Geometry check sheet. Reference: the model listing, model coordinates, mm. A direction names the side the tool comes from. Round coordinates to 2 decimals unless told otherwise and drop trailing zeros. Order: outer loops, then holes, each group sorted by start corner. A loop starts at its lowest first (then second) coordinate and runs counter-clockwise, first axis right, second up.
```python
from build123d import *

# Parameters (mm, degrees)
BOSS_EXTRU_1_DEPTH  = 31.5
ESQUISSE3_R         = 3.5
BOSS_EXTRU_2_DEPTH  = 3
ESQUISSE5_R         = 2
BOSS_EXTRU_3_DEPTH  = 0.5
ESQUISSE6_R         = 2.5
BOSS_EXTRU_4_DEPTH  = 4.5
ESQUISSE8_R         = 2
BOSS_EXTRU_5_DEPTH  = 0.5
ESQUISSE9_R         = 2.5
BOSS_EXTRU_6_DEPTH  = 1
CHANFREIN1_SIZE     = 0.5
ESQUISSE10_R        = 5
BOSS_EXTRU_7_DEPTH  = 2
ESQUISSE11_R        = 3
BOSS_EXTRU_8_DEPTH  = 1
ESQUISSE13_R        = 3.375
BOSS_EXTRU_9_DEPTH  = 5
ESQUISSE15_R        = 3
BOSS_EXTRU_10_DEPTH = 0.5
ESQUISSE16_R        = 3.375
BOSS_EXTRU_11_DEPTH = 6.5


with BuildPart() as part:
    # Esquisse1 → Boss.-Extru.1 (new body)
    with BuildSketch(Plane(origin=(0, 0, 0), x_dir=(1, 0, 0), z_dir=(0, 1, 0))):
        with BuildLine():
            Line((1.18016373, -3.5), (1.18016373, -7.912472027))
            ThreePointArc((1.18016373, -7.912472027), (5.676756903, -5.636881324), (7.920594452, -1.124359161))
            Line((7.920594452, -1.124359161), (3.5, -1.124359161))
            Line((3.5, -1.124359161), (3.5, 1.18016373))
            Line((3.5, 1.18016373), (7.912472027, 1.18016373))
            ThreePointArc((7.912472027, 1.18016373), (5.636881324, 5.676756903), (1.124359161, 7.920594452))
            Line((1.124359161, 7.920594452), (1.124359161, 3.5))
            Line((1.124359161, 3.5), (-1.18016373, 3.5))
            Line((-1.18016373, 3.5), (-1.18016373, 7.912472027))
            ThreePointArc((-1.18016373, 7.912472027), (-5.676756903, 5.636881324), (-7.920594452, 1.124359161))
            Line((-7.920594452, 1.124359161), (-3.5, 1.124359161))
            Line((-3.5, 1.124359161), (-3.5, -1.18016373))
            Line((-3.5, -1.18016373), (-7.912472027, -1.18016373))
            ThreePointArc((-7.912472027, -1.18016373), (-5.636881324, -5.676756903), (-1.124359161, -7.920594452))
            Line((-1.124359161, -7.920594452), (-1.124359161, -3.5))
            Line((-1.124359161, -3.5), (1.18016373, -3.5))
        make_face()
    extrude(amount=BOSS_EXTRU_1_DEPTH)

    # Esquisse3 → Boss.-Extru.2 (add)
    with BuildSketch(Plane.XZ):
        with Locations(Location((0, 0, 0), (0, 0, 270))):
            Circle(ESQUISSE3_R)
    extrude(amount=BOSS_EXTRU_2_DEPTH)

    # Esquisse5 → Boss.-Extru.3 (add)
    with BuildSketch(Plane.XZ.offset(3)):
        with Locations(Location((0, 0, 0), (0, 0, 270))):
            Circle(ESQUISSE5_R)
    extrude(amount=BOSS_EXTRU_3_DEPTH)

    # Esquisse6 → Boss.-Extru.4 (add)
    with BuildSketch(Plane.XZ.offset(3.5)):
        with Locations(Location((0, 0, 0), (0, 0, 270))):
            Circle(ESQUISSE6_R)
    extrude(amount=BOSS_EXTRU_4_DEPTH)

    # Esquisse8 → Boss.-Extru.5 (add)
    with BuildSketch(Plane.XZ.offset(8)):
        with Locations(Location((0, 0, 0), (0, 0, 270))):
            Circle(ESQUISSE8_R)
    extrude(amount=BOSS_EXTRU_5_DEPTH)

    # Esquisse9 → Boss.-Extru.6 (add)
    with BuildSketch(Plane.XZ.offset(8.5)):
        with Locations(Location((0, 0, 0), (0, 0, 270))):
            Circle(ESQUISSE9_R)
    extrude(amount=BOSS_EXTRU_6_DEPTH)

    # Chanfrein1
    chanfrein1_edges = [part.edges().sort_by_distance(p)[0] for p in [
        (0, -9.5, 2.5),
    ]]
    chamfer(chanfrein1_edges, length=CHANFREIN1_SIZE)

    # Esquisse10 → Boss.-Extru.7 (add)
    with BuildSketch(Plane(origin=(0, 31.5, 0), x_dir=(1, 0, 0), z_dir=(0, 1, 0))):
        with Locations(Location((0, 0, 0), (0, 0, 77.004658444))):
            Circle(ESQUISSE10_R)
    extrude(amount=BOSS_EXTRU_7_DEPTH)

    # Esquisse11 → Boss.-Extru.8 (add)
    with BuildSketch(Plane(origin=(0, 33.5, 0), x_dir=(1, 0, 0), z_dir=(0, 1, 0))):
        with Locations(Location((0, 0, 0), (0, 0, 270))):
            Circle(ESQUISSE11_R)
    extrude(amount=BOSS_EXTRU_8_DEPTH)

    # Esquisse13 → Boss.-Extru.9 (add)
    with BuildSketch(Plane(origin=(0, 34.5, 0), x_dir=(1, 0, 0), z_dir=(0, 1, 0))):
        with Locations(Location((0, 0, 0), (0, 0, 270))):
            Circle(ESQUISSE13_R)
    extrude(amount=BOSS_EXTRU_9_DEPTH)

    # Esquisse15 → Boss.-Extru.10 (add)
    with BuildSketch(Plane(origin=(0, 39.5, 0), x_dir=(1, 0, 0), z_dir=(0, 1, 0))):
        with Locations(Location((0, 0, 0), (0, 0, 270))):
            Circle(ESQUISSE15_R)
    extrude(amount=BOSS_EXTRU_10_DEPTH)

    # Esquisse16 → Boss.-Extru.11 (add)
    with BuildSketch(Plane(origin=(0, 40, 0), x_dir=(1, 0, 0), z_dir=(0, 1, 0))):
        with Locations(Location((0, 0, 0), (0, 0, 270))):
            Circle(ESQUISSE16_R)
    extrude(amount=BOSS_EXTRU_11_DEPTH)


solid = part.part
```
(1) Sectioned sample at A-A, the plane z = 5.5. Record the cut outline in (x, y), and give its area (3 significant figures).
Returned:
outline: (-5.81, 0) - (-1.12, 0) - (-1.12, 31.5) - (-5.81, 31.5) - close; (1.18, 0) - (5.81, 0) - (5.81, 31.5) - (1.18, 31.5) - close
area: 293 mm2
(2) Sectioned sample at D-D, the plane y = 42. Record the cut outline in (x, z) (3 decimals), and give its area (3 significant figures).
Returned:
outline: circle Ø6.75 at (0, 0)
area: 35.8 mm2
(3) Depth check by flat-ended pin: P1, Ø5, axis at x = -2.5, z = 5, coming from the -Y side; P2, Ø1.8, axis at y = 19, z = 0, coming from the +X side; P3, Ø1.2, axis at x = 4.5, z = 0, coming from the -Y side. Enter the tip coordinate at first touch or a pass-through.
Returned:
P1: stops at y = -3
P2: stops at x = 3.5
P3: stops at y = 31.5
(4) Draft check along Y on faces 5 (the flat face through (2, -3.5, 1)), 6 (the cylindrical face through (-2.44, -5.72, 0.54)), 7 (the flat face through (0, 46.5, 0)), 8 (the flat face through (4, 0, -4)). Enter one of: released by +Y, released by -Y, zero draft, split by the parting line, or undercut.
Returned:
face 5: undercut
face 6: zero draft
face 7: released by +Y
face 8: released by -Y
(5) Sectioned sample at B-B, the plane y = 22.5. Record the cut outline in (x, z).
Returned:
outline: (-7.92, -1.12) arc R8 ccw to (-1.18, -7.91) - (-1.18, -3.5) - (1.12, -3.5) - (1.12, -7.92) arc R8 ccw to (7.91, -1.18) - (3.5, -1.18) - (3.5, 1.12) - (7.92, 1.12) arc R8 ccw to (1.18, 7.91) - (1.18, 3.5) - (-1.12, 3.5) - (-1.12, 7.92) arc R8 ccw to (-7.91, 1.18) - (-3.5, 1.18) - (-3.5, -1.12) - close
(6) Material ranges on line 1 (Z direction, x = 0.25, y = 11); line 2 (Y direction, x = -2.5, z = 5); line 3 (X direction, y = 7, z = 5) (3 decimals), recorded low to high.
Returned:
line 1: z = -3.5 to 3.5
line 2: y = 0 to 31.5
line 3: x = -6.245 to -1.124, 1.18 to 6.245
(7) Set-up check for faces 1 (the flat face through (2, -8, 1)), 2 (the flat face through (-3.5, 16, 0)), 3 (the flat face through (1.124, 16, -6)), 4 (the flat face through (-4, 0, -4)): record each of +Z, -Z, +X, -X, +Y, -Y from which the full face is reachable in a straight line by a thin tool's end or side.
Returned:
face 1: none
face 2: -X, -Y
face 3: -Z, -Y
face 4: -Z, -X, -Y
(8) Sectioned sample at C-C, the plane x = 6.5. Record the cut outline in (y, z), and give its area (3 significant figures).
Returned:
outline: (0, -4.66) - (31.5, -4.66) - (31.5, -1.18) - (0, -1.18) - close; (0, 1.12) - (31.5, 1.12) - (31.5, 4.66) - (0, 4.66) - close
area: 221 mm2
